Check sheet for the modelled part. Datum: model origin and axes. Units: mm. Face numbers are marked on the shaded views. A direction names the side the tool comes from. Round coordinates to 2 decimals unless told otherwise and drop trailing zeros. Write each loop counter-clockwise with the first axis right and the second up, starting at its lowest first coordinate (ties: lowest second). Pieces come first, ordered by that corner, then holes. Notation, with made-up numbers: (19, 84.5) -> (52, 84.5) arc R21 ccw to (52, 104.5) -> close; hole circle Ø1 at (89.5, -38.75). An arc over 180 degrees is marked (long way). One line per item, written item: value.
from build123d import *

# Parameters (mm, degrees)
SKETCH1_W                    = 44
SKETCH1_H                    = 34.5
SKETCH1_R                    = 1.75
BASE_FLANGE1_DEPTH           = 3.175
EDGE_FLANGE1_STRIP_W         = 16.51
EDGE_FLANGE1_STRIP_H         = 3.175
EDGE_FLANGE1_STRIP_CUT_DEPTH = 44
EDGE_FLANGE1_DEPTH           = 44
EDGE_FLANGE2_STRIP_W         = 16.51
EDGE_FLANGE2_STRIP_H         = 3.175
EDGE_FLANGE2_STRIP_CUT_DEPTH = 44
EDGE_FLANGE2_DEPTH           = 44
CUT_EXTRUDE1_REACH           = 70.083
SKETCH12_R                   = 11.25
SKETCH12_R_2                 = 1.6
CUT_EXTRUDE2_REACH           = 70.083
CHAMFER1_SIZE                = 5
SKETCH14_W                   = 8.7
SKETCH14_H                   = 10
SKETCH14_R                   = 1.6
SKETCH14_W_2                 = 13.3
BOSS_EXTRUDE1_DEPTH          = 3.175
FILLET2_R                    = 5
FILLET3_R                    = 4
BOSS_EXTRUDE3_START          = -3.175
BOSS_EXTRUDE3_DEPTH          = 3.175


# Sheet-metal steps are written as plain solids
with BuildPart() as part:
    # Sketch1 → Base-Flange1 (new body)
    with BuildSketch(Plane(origin=(0, 0, 0), x_dir=(1, 0, 0), z_dir=(0, 1, 0))):
        with Locations((0, 0.25)):
            Rectangle(SKETCH1_W, SKETCH1_H)
        with Locations(Location((-10, 10, 0), (0, 0, 270))):
            Circle(SKETCH1_R, mode=Mode.SUBTRACT)
        with Locations(Location((10, 10, 0), (0, 0, 270))):
            Circle(SKETCH1_R, mode=Mode.SUBTRACT)
        with Locations(Location((10, -10, 0), (0, 0, 270))):
            Circle(SKETCH1_R, mode=Mode.SUBTRACT)
        with Locations(Location((-10, -10, 0), (0, 0, 270))):
            Circle(SKETCH1_R, mode=Mode.SUBTRACT)
    extrude(amount=-BASE_FLANGE1_DEPTH)

    # Edge-Flange1 strip (across the edge) → Edge-Flange1 strip cut (cut)
    with BuildSketch(Plane(origin=(22, 0, -17.5), x_dir=(0, 0, 1), z_dir=(-1, 0, 0))):
        with Locations((-6.35, -1.5875)):
            Rectangle(EDGE_FLANGE1_STRIP_W, EDGE_FLANGE1_STRIP_H)
    extrude(amount=EDGE_FLANGE1_STRIP_CUT_DEPTH, mode=Mode.SUBTRACT)

    # Edge-Flange1 section (across the edge) → Edge-Flange1 (add)
    with BuildSketch(Plane(origin=(22, 0, -17.5), x_dir=(0, 0, 1), z_dir=(-1, 0, 0))):
        with BuildLine():
            Line((-3.175, 1.905), (-3.175, 49.825))
            Line((-3.175, 49.825), (0, 49.825))
            Line((0, 49.825), (0, 1.905))
            ThreePointArc((0, 1.905), (0.557961582, 0.557961582), (1.905, 0))
            Line((1.905, 0), (1.905, -3.175))
            ThreePointArc((1.905, -3.175), (-1.687102448, -1.687102448), (-3.175, 1.905))
        make_face()
    extrude(amount=EDGE_FLANGE1_DEPTH)

    # Edge-Flange2 strip (across the edge) → Edge-Flange2 strip cut (cut)
    with BuildSketch(Plane(origin=(22, -3.175, 17), x_dir=(0, 0, -1), z_dir=(-1, 0, 0))):
        with Locations((-6.35, -1.5875)):
            Rectangle(EDGE_FLANGE2_STRIP_W, EDGE_FLANGE2_STRIP_H)
    extrude(amount=EDGE_FLANGE2_STRIP_CUT_DEPTH, mode=Mode.SUBTRACT)

    # Edge-Flange2 section (across the edge) → Edge-Flange2 (add)
    with BuildSketch(Plane(origin=(22, -3.175, 17), x_dir=(0, 0, -1), z_dir=(-1, 0, 0))):
        with BuildLine():
            Line((-3.175, 1.905), (-3.175, 31.825))
            Line((-3.175, 31.825), (0, 31.825))
            Line((0, 31.825), (0, 1.905))
            ThreePointArc((0, 1.905), (0.557961582, 0.557961582), (1.905, 0))
            Line((1.905, 0), (1.905, -3.175))
            ThreePointArc((1.905, -3.175), (-1.687102448, -1.687102448), (-3.175, 1.905))
        make_face()
    extrude(amount=EDGE_FLANGE2_DEPTH)

    # Sketch12 → Cut-Extrude1 (cut, up to next)
    with BuildSketch(Plane(origin=(0, 0, -20.675), x_dir=(-1, 0, 0), z_dir=(0, 0, -1)), mode=Mode.PRIVATE) as cut_extrude1_sk1:
        with Locations(Location((0, 28, 0), (0, 0, 90))):
            Circle(SKETCH12_R)
    cut_extrude1_tool1 = extrude(cut_extrude1_sk1.sketch, amount=-CUT_EXTRUDE1_REACH, mode=Mode.PRIVATE) & part.part
    # Sketch12 → Cut-Extrude1 (cut, up to next)
    with BuildSketch(Plane(origin=(0, 0, -20.675), x_dir=(-1, 0, 0), z_dir=(0, 0, -1)), mode=Mode.PRIVATE) as cut_extrude1_sk2:
        with Locations(Location((15.5, 43.5, 0), (0, 0, 90))):
            Circle(SKETCH12_R_2)
    cut_extrude1_tool2 = extrude(cut_extrude1_sk2.sketch, amount=-CUT_EXTRUDE1_REACH, mode=Mode.PRIVATE) & part.part
    # Sketch12 → Cut-Extrude1 (cut, up to next)
    with BuildSketch(Plane(origin=(0, 0, -20.675), x_dir=(-1, 0, 0), z_dir=(0, 0, -1)), mode=Mode.PRIVATE) as cut_extrude1_sk3:
        with Locations(Location((15.5, 12.5, 0), (0, 0, 90))):
            Circle(SKETCH12_R_2)
    cut_extrude1_tool3 = extrude(cut_extrude1_sk3.sketch, amount=-CUT_EXTRUDE1_REACH, mode=Mode.PRIVATE) & part.part
    # Sketch12 → Cut-Extrude1 (cut, up to next)
    with BuildSketch(Plane(origin=(0, 0, -20.675), x_dir=(-1, 0, 0), z_dir=(0, 0, -1)), mode=Mode.PRIVATE) as cut_extrude1_sk4:
        with Locations(Location((-15.5, 12.5, 0), (0, 0, 90))):
            Circle(SKETCH12_R_2)
    cut_extrude1_tool4 = extrude(cut_extrude1_sk4.sketch, amount=-CUT_EXTRUDE1_REACH, mode=Mode.PRIVATE) & part.part
    # Sketch12 → Cut-Extrude1 (cut, up to next)
    with BuildSketch(Plane(origin=(0, 0, -20.675), x_dir=(-1, 0, 0), z_dir=(0, 0, -1)), mode=Mode.PRIVATE) as cut_extrude1_sk5:
        with Locations(Location((-15.5, 43.5, 0), (0, 0, 90))):
            Circle(SKETCH12_R_2)
    cut_extrude1_tool5 = extrude(cut_extrude1_sk5.sketch, amount=-CUT_EXTRUDE1_REACH, mode=Mode.PRIVATE) & part.part
    add(cut_extrude1_tool1.solids().sort_by_distance((0, 28, -20.675))[0], mode=Mode.SUBTRACT)
    add(cut_extrude1_tool2.solids().sort_by_distance((-15.5, 43.5, -20.675))[0], mode=Mode.SUBTRACT)
    add(cut_extrude1_tool3.solids().sort_by_distance((-15.5, 12.5, -20.675))[0], mode=Mode.SUBTRACT)
    add(cut_extrude1_tool4.solids().sort_by_distance((15.5, 12.5, -20.675))[0], mode=Mode.SUBTRACT)
    add(cut_extrude1_tool5.solids().sort_by_distance((15.5, 43.5, -20.675))[0], mode=Mode.SUBTRACT)

    # Sketch13 → Cut-Extrude2 (cut, up to next)
    with BuildSketch(Plane.XY.offset(20.175), mode=Mode.PRIVATE) as cut_extrude2_sk1:
        with BuildLine():
            Line((-6.75, -30.175), (-6.75, -24.175))
            ThreePointArc((-6.75, -24.175), (-5, -22.425), (-3.25, -24.175))
            Line((-3.25, -24.175), (-3.25, -30.175))
            ThreePointArc((-3.25, -30.175), (-5, -31.925), (-6.75, -30.175))
        make_face()
    cut_extrude2_tool1 = extrude(cut_extrude2_sk1.sketch, amount=-CUT_EXTRUDE2_REACH, mode=Mode.PRIVATE) & part.part
    # Sketch13 → Cut-Extrude2 (cut, up to next)
    with BuildSketch(Plane.XY.offset(20.175), mode=Mode.PRIVATE) as cut_extrude2_sk2:
        with BuildLine():
            Line((-16.75, -30.175), (-16.75, -24.175))
            ThreePointArc((-16.75, -24.175), (-15, -22.425), (-13.25, -24.175))
            Line((-13.25, -24.175), (-13.25, -30.175))
            ThreePointArc((-13.25, -30.175), (-15, -31.925), (-16.75, -30.175))
        make_face()
    cut_extrude2_tool2 = extrude(cut_extrude2_sk2.sketch, amount=-CUT_EXTRUDE2_REACH, mode=Mode.PRIVATE) & part.part
    # Sketch13 → Cut-Extrude2 (cut, up to next)
    with BuildSketch(Plane.XY.offset(20.175), mode=Mode.PRIVATE) as cut_extrude2_sk3:
        with BuildLine():
            Line((16.75, -30.175), (16.75, -24.175))
            ThreePointArc((16.75, -24.175), (15, -22.425), (13.25, -24.175))
            Line((13.25, -24.175), (13.25, -30.175))
            ThreePointArc((13.25, -30.175), (15, -31.925), (16.75, -30.175))
        make_face()
    cut_extrude2_tool3 = extrude(cut_extrude2_sk3.sketch, amount=-CUT_EXTRUDE2_REACH, mode=Mode.PRIVATE) & part.part
    # Sketch13 → Cut-Extrude2 (cut, up to next)
    with BuildSketch(Plane.XY.offset(20.175), mode=Mode.PRIVATE) as cut_extrude2_sk4:
        with BuildLine():
            Line((6.75, -30.175), (6.75, -24.175))
            ThreePointArc((6.75, -24.175), (5, -22.425), (3.25, -24.175))
            Line((3.25, -24.175), (3.25, -30.175))
            ThreePointArc((3.25, -30.175), (5, -31.925), (6.75, -30.175))
        make_face()
    cut_extrude2_tool4 = extrude(cut_extrude2_sk4.sketch, amount=-CUT_EXTRUDE2_REACH, mode=Mode.PRIVATE) & part.part
    add(cut_extrude2_tool1.solids().sort_by_distance((-5, -27.175, 20.175))[0], mode=Mode.SUBTRACT)
    add(cut_extrude2_tool2.solids().sort_by_distance((-15, -27.175, 20.175))[0], mode=Mode.SUBTRACT)
    add(cut_extrude2_tool3.solids().sort_by_distance((15, -27.175, 20.175))[0], mode=Mode.SUBTRACT)
    add(cut_extrude2_tool4.solids().sort_by_distance((5, -27.175, 20.175))[0], mode=Mode.SUBTRACT)

    # Chamfer1
    chamfer1_edges = [part.edges().sort_by_distance(p)[0] for p in [
        (22, -35, 18.5875),
        (-22, -35, 18.5875),
    ]]
    chamfer(chamfer1_edges, length=CHAMFER1_SIZE)

    # Sketch14 → Boss-Extrude1 (add)
    # profile 1 of 2: a face of its own
    with BuildSketch(Plane(origin=(0, 0, -20.675), x_dir=(-1, 0, 0), z_dir=(0, 0, -1))):
        with Locations((-26.35, 12.85)):
            Rectangle(SKETCH14_W, SKETCH14_H)
        with Locations(Location((-25.7, 12.85, 0), (0, 0, 90))):
            Circle(SKETCH14_R, mode=Mode.SUBTRACT)
    # profile 2 of 2: a face of its own
    with BuildSketch(Plane(origin=(0, 0, -20.675), x_dir=(-1, 0, 0), z_dir=(0, 0, -1))):
        with Locations((28.65, 12.85)):
            Rectangle(SKETCH14_W_2, SKETCH14_H)
        with Locations(Location((30.3, 12.85, 0), (0, 0, 90))):
            Circle(SKETCH14_R, mode=Mode.SUBTRACT)
    extrude(amount=-BOSS_EXTRUDE1_DEPTH)

    # Fillet2
    fillet2_edges = [part.edges().sort_by_distance(p)[0] for p in [
        (-22, 17.85, -19.0875),
        (22, 17.85, -19.0875),
    ]]
    fillet(fillet2_edges, radius=FILLET2_R)

    # Fillet3
    fillet3_edges = [part.edges().sort_by_distance(p)[0] for p in [
        (-35.3, 7.85, -19.0875),
        (-35.3, 17.85, -19.0875),
        (30.7, 7.85, -19.0875),
        (30.7, 17.85, -19.0875),
        (-22, 49.825, -19.0875),
        (22, 49.825, -19.0875),
        (-22, 7.85, -19.0875),
        (22, 7.85, -19.0875),
        (-22, -30, 18.5875),
        (-17, -35, 18.5875),
        (17, -35, 18.5875),
        (22, -30, 18.5875),
    ]]
    fillet(fillet3_edges, radius=FILLET3_R)

    # Sketch19 → Boss-Extrude3 (add)
    with BuildSketch(Plane(origin=(0, 0, -20.675), x_dir=(-1, 0, 0), z_dir=(0, 0, -1)).offset(BOSS_EXTRUDE3_START)):
        with BuildLine():
            ThreePointArc((-25.2, 34.5), (-23.6, 36.1), (-22, 34.5))
            Line((-22, 34.5), (-22, 41.588723439))
            ThreePointArc((-22, 41.588723439), (-22.546495251, 40.214924348), (-23.887323944, 39.591899935))
            ThreePointArc((-23.887323944, 39.591899935), (-27.306437111, 38.003187683), (-28.7, 34.5))
            Line((-28.7, 34.5), (-28.7, 29.5))
            ThreePointArc((-28.7, 29.5), (-27.314329906, 26.005181929), (-23.910292804, 24.409448127))
            ThreePointArc((-23.910292804, 24.409448127), (-22.479211599, 23.673677736), (-22.053293762, 22.121922124))
            ThreePointArc((-22.053293762, 22.121922124), (-22.013341239, 22.484987117), (-22, 22.85))
            Line((-22, 22.85), (-22, 29.5))
            ThreePointArc((-22, 29.5), (-23.6, 27.9), (-25.2, 29.5))
            Line((-25.2, 29.5), (-25.2, 34.5))
        make_face()
    extrude(amount=BOSS_EXTRUDE3_DEPTH)


solid = part.part
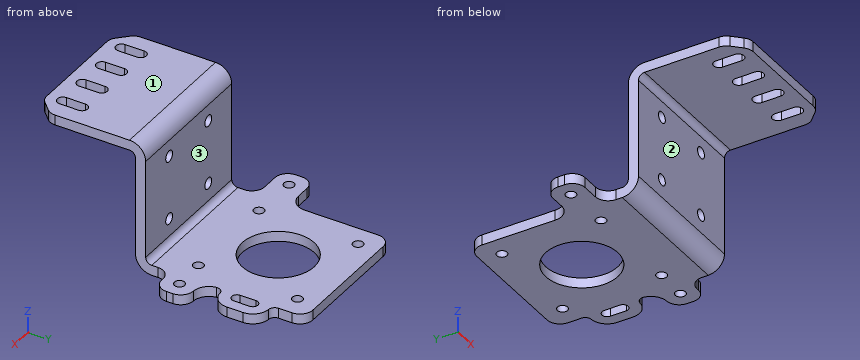
Item 1: Depth check by flat-ended pin: P1, Ø4, axis at x = -15.5, y = 43.5, coming from the +Z side; P2, Ø1, axis at y = -26.5, z = 18, coming from the +X side; P3, Ø1.6, axis at x = -29.5, z = -19.5, coming from the -Y side. Enter the tip coordinate at first touch or a pass-through.
Answer:
P1: stops at z = -17.5
P2: stops at x = 22
P3: stops at y = 7.85
Item 2: Sectioned sample at C-C on z = 0. Enter the section's corners in (x, y) (3 decimals).
Answer:
outline: (-22, -3.175) -> (22, -3.175) -> (22, 0) -> (-22, 0) -> close
Item 3: Sectioned sample at D-D on x = -10. Enter the section's corners in (y, z) (3 decimals), and give its area (3 significant figures).
Answer:
outline: (-35, 17) -> (-5.08, 17) arc R1.905 cw to (-3.175, 15.095) -> (-3.175, 11.75) -> (0, 11.75) -> (0, 15.095) arc R5.08 ccw to (-5.08, 20.175) -> (-35, 20.175) -> close; (-3.175, -15.595) arc R5.08 ccw to (1.905, -20.675) -> (22.846, -20.675) -> (22.846, -17.5) -> (1.905, -17.5) arc R1.905 cw to (0, -15.595) -> (0, -11.75) -> (-3.175, -11.75) -> close; (-3.175, -8.25) -> (0, -8.25) -> (0, 8.25) -> (-3.175, 8.25) -> close; (33.154, -20.675) -> (49.825, -20.675) -> (49.825, -17.5) -> (33.154, -17.5) -> close
area: 324 mm^2
Item 4: Sectioned sample at B-B on y = 20.5. Enter the section's corners in (x, z) (3 decimals), and give its area (3 significant figures).
Answer:
outline: (-22.587, -20.675) -> (-8.385, -20.675) -> (-8.385, -17.5) -> (-22.587, -17.5) -> close; (8.385, -20.675) -> (22.587, -20.675) -> (22.587, -17.5) -> (8.385, -17.5) -> close
area: 90.2 mm^2
Item 5: Thickness scan on line 1 (Y direction, x = -15, z = -18) (3 decimals); line 2 (X direction, y = -1, z = -10); line 3 (X direction, y = 12.5, z = -18.2). Record the ranges inside material, lowest first.
Answer:
line 1: y = -2.57 to 10.98, 14.02 to 41.98, 45.02 to 49.825
line 2: x = -22 to -11.75, -8.25 to 8.25, 11.75 to 22
line 3: x = -35.3 to -31.86, -28.74 to -17.1, -13.9 to 13.9, 17.1 to 24.14, 27.26 to 30.7
Item 6: Tool access check on the marked faces 1, 2 and 3. Record the directions out of +Z, -Z, +X, -X, +Y, -Y that give a thin tool (end or side, any length) a straight path to the whole face; none if there is none.
Answer:
face 1: +Z, +X, -X, +Y, -Y
face 2: -Z, +X, -X, -Y
face 3: +Z, +X, -X, +Y
Item 7: Sectioned sample at A-A on x = 0. Enter the section's corners in (y, z) (3 decimals).
Answer:
outline: (-35, 17) -> (-5.08, 17) arc R1.905 cw to (-3.175, 15.095) -> (-3.175, -15.595) arc R5.08 ccw to (1.905, -20.675) -> (16.75, -20.675) -> (16.75, -17.5) -> (1.905, -17.5) arc R1.905 cw to (0, -15.595) -> (0, 15.095) arc R5.08 ccw to (-5.08, 20.175) -> (-35, 20.175) -> close; (39.25, -20.675) -> (49.825, -20.675) -> (49.825, -17.5) -> (39.25, -17.5) -> close
